```python
from build123d import *

# Parameters (mm, degrees)
SKETCH1_R               = 50.8
BOSS_EXTRUDE1_DEPTH     = 457.2
SKETCH2_R               = 47.625
CUT_EXTRUDE1_DEPTH      = 458.2
SKETCH3_R               = 27.989032433
SKETCH3_W               = 25.4
SKETCH3_H               = 381
CUT_EXTRUDE3_DEPTH      = 51.8
CUT_EXTRUDE3_DEPTH_BACK = 51.8
BOSS_EXTRUDE2_DEPTH     = 381
SKETCH6_R               = 50.8
BOSS_EXTRUDE3_DEPTH     = 50.8
CUT_EXTRUDE4_DEPTH      = 25.4
SKETCH8_R               = 3.302
CUT_EXTRUDE5_DEPTH      = 73.916768016
BOSS_EXTRUDE4_DEPTH     = 2.54
BOSS_EXTRUDE5_DEPTH     = 2.54
SKETCH26_W              = 12.7
SKETCH26_H              = 19.05
CUT_EXTRUDE6_DEPTH      = 84.582


with BuildPart() as part:
    # Sketch1 → Boss-Extrude1 (new body)
    with BuildSketch(Plane(origin=(0, 0, 0), x_dir=(1, 0, 0), z_dir=(0, 1, 0))):
        Circle(SKETCH1_R)
    extrude(amount=BOSS_EXTRUDE1_DEPTH)

    # Sketch2 → Cut-Extrude1 (cut, through all)
    with BuildSketch(Plane(origin=(0, 457.2, 0), x_dir=(1, 0, 0), z_dir=(0, 1, 0))):
        Circle(SKETCH2_R)
    extrude(amount=-CUT_EXTRUDE1_DEPTH, mode=Mode.SUBTRACT)

    # Sketch3 → Cut-Extrude3 (cut, two sides)
    with BuildSketch(Plane.XY) as cut_extrude3_sk:
        with Locations((-12.065, 228.6)):
            Circle(SKETCH3_R)
        with Locations((38.1, 228.6)):
            Rectangle(SKETCH3_W, SKETCH3_H)
    extrude(amount=CUT_EXTRUDE3_DEPTH, mode=Mode.SUBTRACT)
    extrude(cut_extrude3_sk.sketch, amount=-CUT_EXTRUDE3_DEPTH_BACK, mode=Mode.SUBTRACT)

    # Sketch5 → Boss-Extrude2 (add)
    with BuildSketch(Plane(origin=(0, 38.1, 0), x_dir=(1, 0, 0), z_dir=(0, 1, 0))):
        Polygon((25.4, -43.994090512), (25.4, 43.994090512), (27.573729132, 42.665319192), (27.573729132, -42.665319192), align=None)
    extrude(amount=BOSS_EXTRUDE2_DEPTH)

    # Sketch6 → Boss-Extrude3 (add)
    with BuildSketch(Plane.XZ):
        Circle(SKETCH6_R)
    extrude(amount=BOSS_EXTRUDE3_DEPTH)

    # Sketch7 → Cut-Extrude4 (cut)
    with BuildSketch(Plane.XZ.offset(50.8)):
        with BuildLine():
            Line((17.374623281, 47.736385136), (17.374623281, 22.116767912))
            Line((17.374623281, 22.116767912), (-17.374623281, 22.116767912))
            Line((-17.374623281, 22.116767912), (-17.374623281, 47.736385136))
            ThreePointArc((-17.374623281, 47.736385136), (-8.821327425, 50.028233853), (0, 50.8))
            ThreePointArc((0, 50.8), (8.821327425, 50.028233853), (17.374623281, 47.736385136))
        make_face()
        with BuildLine():
            Line((17.374623281, -22.116767912), (-17.374623281, -22.116767912))
            Line((-17.374623281, -22.116767912), (-17.374623281, -47.736385136))
            ThreePointArc((-17.374623281, -47.736385136), (-8.821327425, -50.028233853), (0, -50.8))
            ThreePointArc((0, -50.8), (8.821327425, -50.028233853), (17.374623281, -47.736385136))
            Line((17.374623281, -47.736385136), (17.374623281, -22.116767912))
        make_face()
    extrude(amount=-CUT_EXTRUDE4_DEPTH, mode=Mode.SUBTRACT)

    # Sketch8 → Cut-Extrude5 (cut, through all)
    with BuildSketch(Plane.XY.offset(22.116767912)):
        with Locations((0, -38.091466754)):
            Circle(SKETCH8_R)
    extrude(amount=-CUT_EXTRUDE5_DEPTH, mode=Mode.SUBTRACT)

    # Sketch9 → Boss-Extrude4 (add)
    with BuildSketch(Plane(origin=(0, 38.1, 0), x_dir=(1, 0, 0), z_dir=(0, 1, 0))):
        with BuildLine():
            Line((27.573729132, 42.665319192), (27.573729132, -42.665319192))
            ThreePointArc((27.573729132, -42.665319192), (50.8, 0), (27.573729132, 42.665319192))
        make_face()
    extrude(amount=BOSS_EXTRUDE4_DEPTH)

    # Sketch10 → Boss-Extrude5 (add)
    with BuildSketch(Plane.XZ.offset(-419.1)):
        with BuildLine():
            Line((27.573729132, 42.665319192), (27.573729132, -42.665319192))
            ThreePointArc((27.573729132, -42.665319192), (50.8, 0), (27.573729132, 42.665319192))
        make_face()
    extrude(amount=BOSS_EXTRUDE5_DEPTH)

    # Sketch26 → Cut-Extrude6 (cut)
    with BuildSketch(Plane.XZ.offset(50.8)):
        Rectangle(SKETCH26_W, SKETCH26_H)
    extrude(amount=-CUT_EXTRUDE6_DEPTH, mode=Mode.SUBTRACT)


solid = part.part
```
Build history of the part. All positions in model axes, mm. A direction names the side the tool comes from. Round coordinates to 2 decimals unless told otherwise and drop trailing zeros. Write each loop counter-clockwise with the first axis right and the second up, starting at its lowest first coordinate (ties: lowest second). Pieces come first, ordered by that corner, then holes.
1) Pin check, flat tips, straight feed: pin 1 (2 mm diameter, centred on y = 0.5, z = -22, fed in from -X); pin 2 (20.5 mm diameter, centred on y = -32.5, z = 40, fed in from -X); pin 3 (4 mm diameter, centred on y = 245, z = 3.5, fed in from -X). Stop position of each tip, or through.
2) Band-saw the part on C-C, the plane y = 228.6. List the corners of the cut face in (x, z) (3 decimals).
3) Band-saw the part on A-A, the plane z = 0. List the corners of the cut face in (x, y) (3 decimals), and give its area (3 significant figures).
4) 3-axis set-ups, long thin cutter, end or side, ignore diameter. For faces 4 (the flat face through (0, -26, -9.525)), 5 (the flat face through (36, 416.56, 1)), 6 (the flat face through (17.375, -38, 35)), 7 (the flat face through (34, 38.1, -1)), 8 (the flat face through (4, -38, -22.117)): which of +Z, -Z, +X, -X, +Y, -Y reach the whole face in a straight line?
5) Band-saw the part on B-B, the plane y = 397. List the corners of the cut face in (x, z) (3 decimals), and give its area (3 significant figures).
6) Drill centre lines: probe 1 along Y at (x, z) = (26, 19.5); probe 2 along Y at (x, z) = (0, -19); probe 3 along Z at (x, y) = (3, 96.5). Where is each one in solid material? Low to high.
7) Band-saw the part on D-D, the plane x = 11.5. List the corners of the cut face in (y, z).
8) Mould opens along Y. For faces 1 (the flat face through (36, 40.64, -1)), 2 (the flat face through (-15.3, 457.2, -45.4)), 3 (the flat face through (-17.375, -38, 35)) say: +Y half, -Y half, draft (parallel to the pull), parting line (faces both ways), or undercut.
Ans:
1. pin 1: stops at x = -46.26
1. pin 2: stops at x = -41.18
1. pin 3: stops at x = -50.78
2. outline: (-40.054, -31.246) - (-40.054, -25.765) arc R47.625 cw to (-40.054, 25.765) - (-40.054, 31.246) arc R50.8 ccw to start; (15.924, -48.24) arc R50.8 ccw to (25.4, -43.994) - (27.574, -42.665) - (27.574, 42.665) - (25.4, 43.994) arc R50.8 ccw to (15.924, 48.24) - (15.924, 44.884) arc R47.625 cw to (25.4, 40.286) - (25.4, -40.286) arc R47.625 cw to (15.924, -44.884) - close
3. outline: (-50.8, -50.8) - (-6.35, -50.8) - (-6.35, 0) - (-47.625, 0) - (-47.625, 457.2) - (-50.8, 457.2) - close; (6.35, -50.8) - (50.8, -50.8) - (50.8, 40.64) - (27.574, 40.64) - (27.574, 416.56) - (50.8, 416.56) - (50.8, 457.2) - (47.625, 457.2) - (47.625, 419.1) - (25.4, 419.1) - (25.4, 38.1) - (47.625, 38.1) - (47.625, 0) - (6.35, 0) - close
3. area: 7,160 mm2
4. face 4: +Y, -Y
4. face 5: +Z, -Z, +X
4. face 6: +Z, -Y
4. face 7: none
4. face 8: -Z, -Y
5. outline: (25.4, -43.994) - (27.574, -42.665) - (27.574, 42.665) - (25.4, 43.994) arc R50.8 ccw (long way) to start; hole (25.4, -40.286) - (25.4, 40.286) arc R47.625 ccw (long way) to start
5. area: 849 mm2
6. probe 1: y = -50.8 to 0, 38.1 to 419.1
6. probe 2: y = -50.8 to -41.39, -34.79 to 0
6. probe 3: z = -50.71 to -47.53, 47.53 to 50.71
7. outline: (-50.8, -22.12) - (-25.4, -22.12) - (-25.4, -49.48) - (213.5, -49.48) - (213.5, -46.22) - (0, -46.22) - (0, 46.22) - (213.5, 46.22) - (213.5, 49.48) - (-25.4, 49.48) - (-25.4, 22.12) - (-50.8, 22.12) - close; (243.7, -49.48) - (457.2, -49.48) - (457.2, -46.22) - (243.7, -46.22) - close; (243.7, 46.22) - (457.2, 46.22) - (457.2, 49.48) - (243.7, 49.48) - close
8. face 1: undercut
8. face 2: +Y half
8. face 3: draft
